Autodesk Inventor part; units mm, degrees
ref_plane "dummy_XY" through (0, 0, 0) normal (1, 0, 0) x (0, 0, -1)
ref_plane "dummy_YZ" through (0, 0, 0) normal (0, 0, -1) x (0, 1, 0)
ref_plane "dummy_ZX" through (0, 0, 0) normal (0, 1, 0) x (1, 0, 0)
sketch "Sketch_1" plane through (0, 0, 0) normal (1, 0, 0) x (0, 1, 0)
  line L0 (4.25, 7.5) -> (-4.25, 7.5)
  arc A0 (-4.25, 7.5) -> (-5, 6.75) centre (-4.25, 6.75) ccw
  line L1 (-5, 6.75) -> (-5, -6.75)
  arc A1 (-5, -6.75) -> (-4.25, -7.5) centre (-4.25, -6.75) ccw
  line L2 (-4.25, -7.5) -> (4.25, -7.5)
  arc A2 (4.25, -7.5) -> (5, -6.75) centre (4.25, -6.75) ccw
  line L3 (5, -6.75) -> (5, 6.75)
  arc A3 (5, 6.75) -> (4.25, 7.5) centre (4.25, 6.75) ccw
extrude "Extrusion1" add sketch "Sketch_1" against normal blind 3
sketch "Sketch_2" plane through (0, 0, 0) normal (0, 0, 1) x (1, 0, 0)
  line L0 (3, 0) -> (-3, 0)
  line L1 (-4.6, 3.45) -> (-1.6, 3.45)
  line L2 (-1.6, 3.45) -> (-1.6, 13.45)
  line L3 (-1.6, 13.45) -> (-4.6, 13.45)
  line L4 (-4.6, 13.45) -> (-4.6, 3.45)
revolve "Revolution1" cut sketch "Sketch_2" angle 360 about axis through (3, 0, 0) along (1, 0, 0)
sketch "Sketch_3" plane through (0, 0, 0) normal (0, 0, 1) x (1, 0, 0)
  line L0 (0, 0) -> (-3, 0)
  line L1 (-3, 0) -> (-3, 2)
  line L2 (-3, 2) -> (-2.621, 1.621)
  line L3 (-2.621, 1.621) -> (-0.379, 1.621)
  line L4 (-0.379, 1.621) -> (0, 2)
  line L5 (0, 2) -> (0, 0)
  line L6 (0, 0) -> (-3, 0)
revolve "Revolution2" cut sketch "Sketch_3" angle 360 about axis through (0, 0, 0) along (1, 0, 0)
thread "Thread1"
ref_plane "dummy_XY" through (0, 0, 0) normal (1, 0, 0) x (0, 0, -1)
ref_plane "dummy_YZ" through (0, 0, 0) normal (0, 0, -1) x (0, 1, 0)
ref_plane "dummy_ZX" through (0, 0, 0) normal (0, 1, 0) x (1, 0, 0)
properties part number "HNKK5-4" material "Steel, Alloy"
Input: part model. Units: mm. Frame: model coordinates. A direction names the side the tool comes from. Round coordinates to 2 decimals unless told otherwise and drop trailing zeros. Loops run counter-clockwise (first coordinate to the right, second up) from the corner with the lowest first, then second, coordinate; pieces in that order, holes last. Notation, with made-up numbers: (35, 49.25) -> (44, 49.25) arc R5 ccw to (44, 56.25) -> close; hole circle Ø2 at (-3, 58.5). An arc over 180 degrees is marked (long way). Answer as a JSON object with one key per item and string values. Group by question number.
1) Section query B-B on y = 0. Output: boundary loops of the cut face in (x, z), plus the area to 3 significant figures.
2) Ray query, L1, parallel to Z at x = -1.45, y = 0; L2, parallel to Z at x = -1.75, y = 0; L3, parallel to X at y = 4.5, z = 0. Return the intervals inside material, ascending.
3) Section query C-C on x = -0.55. Output: boundary loops of the cut face in (y, z), plus the area to 3 significant figures.
4) Reachability of faces 1 (the flat face through (-3, 0, -2.3)), 2 (the cylindrical face through (-2.29, -0.45, 3.42)) from +Z, -Z, +X, -X, +Y, -Y: full face, straight path, thin tool, end or side. Return the list, or none.
5) Section query A-A on z = 0. Output: boundary loops of the cut face in (x, y).
6) Section query D-D on y = -3. Output: boundary loops of the cut face in (x, z).
7) Draft query along Y for faces 3 (the flat face through (-1, 0, -7.5)), 4 (the cylindrical face through (-1.484, 0.748, -1.438)), 5 (the flat face through (-1, -5, 0)). Return one class per face: +Y half, -Y half, draft (parallel to the pull), parting line (faces both ways), or undercut.
Reply:
{
 "1": {"outline": "(-3, -3.45) -> (-1.6, -3.45) -> (-1.6, -7.5) -> (0, -7.5) -> (0, -2) -> (-0.38, -1.62) -> (-2.62, -1.62) -> (-3, -2) -> close; (-3, 2) -> (-2.62, 1.62) -> (-0.38, 1.62) -> (0, 2) -> (0, 7.5) -> (-1.6, 7.5) -> (-1.6, 3.45) -> (-3, 3.45) -> close", "area": "23.6 mm2"},
 "2": {"L1": "z = -7.5 to -1.62, 1.62 to 7.5", "L2": "z = -3.45 to -1.62, 1.62 to 3.45", "L3": "x = -1.6 to 0"},
 "3": {"outline": "(-5, -6.75) arc R0.75 ccw to (-4.25, -7.5) -> (4.25, -7.5) arc R0.75 ccw to (5, -6.75) -> (5, 6.75) arc R0.75 ccw to (4.25, 7.5) -> (-4.25, 7.5) arc R0.75 ccw to (-5, 6.75) -> close; hole circle Ø3.24 at (0, 0)", "area": "141 mm2"},
 "4": {"face 1": "+Z, -Z, -X, +Y, -Y", "face 2": "-X"},
 "5": {"outline": "(-3, -3.45) -> (-1.6, -3.45) -> (-1.6, -5) -> (0, -5) -> (0, -2) -> (-0.38, -1.62) -> (-2.62, -1.62) -> (-3, -2) -> close; (-3, 2) -> (-2.62, 1.62) -> (-0.38, 1.62) -> (0, 2) -> (0, 5) -> (-1.6, 5) -> (-1.6, 3.45) -> (-3, 3.45) -> close"},
 "6": {"outline": "(-3, -1.7) -> (-1.6, -1.7) -> (-1.6, -7.5) -> (0, -7.5) -> (0, 7.5) -> (-1.6, 7.5) -> (-1.6, 1.7) -> (-3, 1.7) -> close"},
 "7": {"face 3": "draft", "face 4": "undercut", "face 5": "-Y half"}
}
